Part model, mm, in its own coordinate system. Face numbers are marked on the shaded views. A direction names the side the tool comes from. Round coordinates to 2 decimals unless told otherwise and drop trailing zeros. Write each loop counter-clockwise with the first axis right and the second up, starting at its lowest first coordinate (ties: lowest second). Pieces come first, ordered by that corner, then holes.
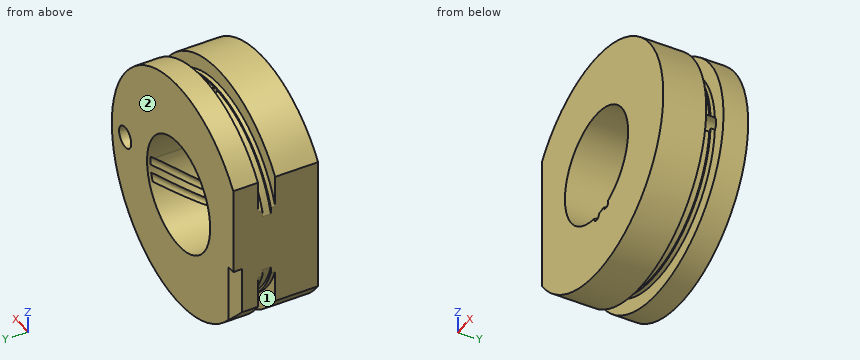
```python
from build123d import *

# Parameters (mm, degrees)
EXTRUDE_1_DEPTH           = 19.75
SKETCH_2_R                = 13
CUT_EXTRUDE_2_DEPTH       = 20.75
CUT_EXTRUDE_4_DEPTH       = 23.69
HOLE_WIZARD_5_0_5_1_D     = 5
HOLE_WIZARD_5_0_5_1_DEPTH = 12
SKETCH_9_R                = 1
CUT_EXTRUDE_5_DEPTH       = 28.5
SWEEP_1_PITCH             = 95
SWEEP_1_HEIGHT            = 19
SWEEP_1_RADIUS            = 13
SWEEP_1_START_ANGLE       = -180
SKETCH_11_R               = 1
PATTERN_CIRCULAR_1_COUNT  = 2
PATTERN_CIRCULAR_1_ANGLE  = 17


with BuildPart() as part:
    # Эскиз1 → Бобышка-Вытянуть1 (new body)
    with BuildSketch(Plane(origin=(0, 0, 0), x_dir=(1, 0, 0), z_dir=(0, 1, 0))):
        with BuildLine():
            Line((-22.5, 15.811388301), (-22.5, -15.811388301))
            ThreePointArc((-22.5, -15.811388301), (27.5, 0), (-22.5, 15.811388301))
        make_face()
    extrude(amount=EXTRUDE_1_DEPTH)

    # Эскиз2 → Вырез-Вытянуть2 (cut, through all)
    with BuildSketch(Plane(origin=(0, 0, 0), x_dir=(1, 0, 0), z_dir=(0, 1, 0))):
        Circle(SKETCH_2_R)
    extrude(amount=CUT_EXTRUDE_2_DEPTH, mode=Mode.SUBTRACT)

    # Эскиз3 → Вырез-Повернуть1 (revolve, cut)
    with BuildSketch(Plane(origin=(0, 0, 0), x_dir=(0, 0, -1), z_dir=(1, 0, 0))):
        Polygon((-29, 14), (-24, 14), (-24, 13), (-23.5, 13), (-23.5, 11), (-24, 11), (-24, 10), (-29, 10), align=None)
    revolve(axis=Axis((0, 0, 0), (0, 1, 0)), mode=Mode.SUBTRACT)

    # Эскиз5 → Вырез-Вытянуть4 (cut, through all)
    with BuildSketch(Plane.XY.offset(-4.81)):
        Polygon((-22.5, 19.75), (-20.5, 19.75), (-22.5, 17.75), align=None)
    extrude(amount=-CUT_EXTRUDE_4_DEPTH, mode=Mode.SUBTRACT)

    # Диаметр отверстия Ø5.0 (5)1
    with Locations(Plane(origin=(0, 19.75, 0), x_dir=(1, 0, 0), z_dir=(0, 1, 0))):
        with Locations((22, 0)):
            Hole(HOLE_WIZARD_5_0_5_1_D / 2, depth=HOLE_WIZARD_5_0_5_1_DEPTH)

    # Эскиз9 → Вырез-Вытянуть5 (cut, through all)
    with BuildSketch(Plane.XY):
        with Locations((0, 12)):
            Circle(SKETCH_9_R)
    extrude(amount=CUT_EXTRUDE_5_DEPTH, mode=Mode.SUBTRACT)

    # Вырез-По траектории1: sweep along a helix
    with BuildLine() as sweep_1_path:
        add(Helix(SWEEP_1_PITCH, SWEEP_1_HEIGHT, SWEEP_1_RADIUS, center=(0, 0, 0), direction=(0, 1, 0), lefthand=True, mode=Mode.PRIVATE).rotate(Axis((0, 0, 0), (0, 1, 0)), SWEEP_1_START_ANGLE))
    # Эскиз11 → Вырез-По траектории1 (sweep, cut)
    with BuildSketch(Plane(origin=(0, 0, 0), x_dir=(1, 0, 0), z_dir=(0, 1, 0))):
        with Locations((0, 13)):
            Circle(SKETCH_11_R)
    sweep_1 = sweep(path=sweep_1_path.line, is_frenet=True, mode=Mode.SUBTRACT)

    # Круговой массив1: Вырез-По траектории1 ×2 about axis
    pattern_circular_1_axis = Axis((0, 19.75, 0), (0, -1, 0))
    for i in range(1, PATTERN_CIRCULAR_1_COUNT):
        add(sweep_1.rotate(pattern_circular_1_axis, i * PATTERN_CIRCULAR_1_ANGLE / (PATTERN_CIRCULAR_1_COUNT - 1)), mode=Mode.SUBTRACT)


solid = part.part
```
Q1. Cut at B-B on z = 22. Write the cut outline in (x, y), plus the area to 3 significant figures.
Values follow:
outline: (-16.5, 0) - (16.5, 0) - (16.5, 10) - (9.59, 10) - (9.59, 11) - (8.26, 11) - (8.26, 13) - (9.59, 13) - (9.59, 14) - (16.5, 14) - (16.5, 19.75) - (-16.5, 19.75) - (-16.5, 14) - (-9.59, 14) - (-9.59, 13) - (-8.26, 13) - (-8.26, 11) - (-9.59, 11) - (-9.59, 10) - (-16.5, 10) - close; hole circle Ø2 at (0, 12)
area: 588 mm2
Q2. Cut at C-C on z = -16.5. Write the cut outline in (x, y), plus the area to 3 significant figures.
Values follow:
outline: (-22, 0) - (22, 0) - (22, 10) - (17.43, 10) - (17.43, 11) - (16.73, 11) - (16.73, 13) - (17.43, 13) - (17.43, 14) - (22, 14) - (22, 19.75) - (-20.5, 19.75) - (-22, 18.25) - (-22, 14) - (-17.43, 14) - (-17.43, 13) - (-16.73, 13) - (-16.73, 11) - (-17.43, 11) - (-17.43, 10) - (-22, 10) - close
area: 829 mm2
Q3. Wall check: L1, parallel to Y at x = 25.5, z = 0; L2, parallel to Z at x = 0, y = 10.5; L3, parallel to Y at x = 0, z = 20. Give the ranges that are in metal, low to high.
Values follow:
L1: y = 0 to 10, 14 to 19.75
L2: z = -24 to -13, 13 to 24
L3: y = 0 to 11, 13 to 19.75
Q4. Cut at D-D on x = 22. Write the cut outline in (y, z).
Values follow:
outline: (0, -16.5) - (10, -16.5) - (10, -9.59) - (11, -9.59) - (11, -8.26) - (13, -8.26) - (13, -9.59) - (14, -9.59) - (14, -16.5) - (19.75, -16.5) - (19.75, -2.5) - (7.75, -2.5) - (7.75, 2.5) - (19.75, 2.5) - (19.75, 16.5) - (14, 16.5) - (14, 9.59) - (13, 9.59) - (13, 8.26) - (11, 8.26) - (11, 9.59) - (10, 9.59) - (10, 16.5) - (0, 16.5) - close
Q5. Cut at A-A on x = -10. Write the cut outline in (y, z).
Values follow:
outline: (0, -25.62) - (10, -25.62) - (10, -21.82) - (11, -21.82) - (11, -21.27) - (13, -21.27) - (13, -21.82) - (14, -21.82) - (14, -25.62) - (19.75, -25.62) - (19.75, -8.31) - (0, -8.31) - close; (0, 8.31) - (19.75, 8.31) - (19.75, 25.62) - (14, 25.62) - (14, 21.82) - (13, 21.82) - (13, 21.27) - (11, 21.27) - (11, 21.82) - (10, 21.82) - (10, 25.62) - (0, 25.62) - close
Q6. Drop flat-ended pins along their axis: pin 1 (2 mm diameter, centred on x = -21.5, y = 19, fed in from -Z); pin 2 (1.8 mm diameter, centred on x = 0, y = 12, fed in from +Z); pin 3 (8 mm diameter, centred on x = 2.5, z = 5.5, fed in from -Y). Give the stop position or say it passes through.
Values follow:
pin 1: stops at z = -18.33
pin 2: stops at z = -12.97
pin 3: passes through
Q7. Which spindle directions (+Z, -Z, +X, -X, +Y, -Y) get a long thin tool onto all of the face, cutting with end or side? Do the marked faces 1 and 2. Say none if no direction does.
Values follow:
face 1: none
face 2: +Z, -Z, +X, -X, +Y
